Autodesk Inventor part; units mm, degrees
ref_plane "WeldJoint" through (0, 0, -10) normal (0.5, -0.866, 0) x (0, 0, 1)
ref_plane "Inlet_Clock_Angle_plane" through (0, 0, -10) normal (0, 1, 0) x (0, 0, 1)
ref_plane "Charging" through (0, 0, -10) normal (1, 0, 0) x (0, 0, 1)
sketch "Sketch13" plane through (0, 0, 0) normal (0, 0, 1) x (1, 0, 0)
  circle A0 centre (0, 0) radius 600 construction
  line L0 (0, 0) -> (0, -600)
  line L1 (0, 0) -> (-519.6152, -300)
  line L2 (0, 0) -> (600, 0)
  line L3 (0, 0) -> (0, -600)
  line L4 (0, 0) -> (0, -600)
  line L5 (0, 0) -> (534.6039, 272.3943)
  line L6 (0, 0) -> (0, 600)
  dimension "d53" = 1200
  dimension "d55" = 0
  dimension "d98" = 180
  dimension "d99" = 240
  dimension "d100" = 63
  dimension "d101" = 90
ref_plane "WeldJoint" through (0, 0, -10) normal (0.5, -0.866, 0) x (0, 0, 1)
ref_plane "Inlet_Clock_Angle_plane" through (0, 0, -10) normal (0, 1, 0) x (0, 0, 1)
ref_plane "Charging" through (0, 0, -10) normal (1, 0, 0) x (0, 0, 1)
ref_plane "Accsess" through (0, 0, -10) normal (1, 0, 0) x (0, 0, 1)
sketch "Sketch14" plane through (0, 0, -10) normal (0.5, -0.866, 0) x (0, 0, 1)
  line L0 (1710, 594) -> (10, 594)
  line L1 (10, 594) -> (10, 600)
  line L2 (10, 600) -> (1710, 600)
  line L3 (1710, 600) -> (1710, 594)
  line L4 (10, 0) -> (1710, 0)
  line L5 (10, 600) -> (-20, 600) construction
  line L6 (10, 594) -> (-20, 594) construction
  arc A0 (-20, 594) -> (-109.2789, 539.0476) centre (-20, 494) ccw construction
  arc A1 (-109.2789, 539.0476) -> (-234, 15) centre (929.3202, 15) ccw construction
  line L7 (-234, 15) -> (-234, 0) construction
  line L8 (10, 0) -> (-234, 0) construction
  arc A2 (-20, 600) -> (-114.6356, 541.7504) centre (-20, 494) ccw construction
  arc A3 (-114.6356, 541.7504) -> (-240, 15) centre (929.3202, 15) ccw construction
  line L9 (-240, 15) -> (-240, 0) construction
  line L10 (-234, 0) -> (-240, 0) construction
  line L11 (1710, 594) -> (1740, 594)
  line L12 (1710, 600) -> (1740, 600)
  line L13 (1710, 0) -> (1954, 0) construction
  line L14 (1960, 0) -> (1960, 15) construction
  arc A4 (1960, 15) -> (1834.6356, 541.7504) centre (790.6798, 15) ccw construction
  arc A5 (1834.6356, 541.7504) -> (1740, 600) centre (1740, 494) ccw construction
  line L15 (1954, 0) -> (1954, 15) construction
  line L16 (1954, 0) -> (1960, 0) construction
  arc A6 (1954, 15) -> (1829.2789, 539.0476) centre (790.6798, 15) ccw construction
  arc A7 (1829.2789, 539.0476) -> (1740, 594) centre (1740, 494) ccw construction
  line L17 (-160.8038, 520) -> (-540, 520)
  line L18 (-540, 520) -> (-540, 440)
  line L19 (-540, 440) -> (-160.8038, 440)
  line L20 (-160.8038, 440) -> (-160.8038, 520)
  line L21 (1960, 15) -> (1990, 15) construction
  line L22 (1990, 15) -> (1990, 0) construction
  line L23 (1990, 0) -> (1960, 0) construction
  line L24 (-540, 600) -> (-540, 520)
  line L25 (-540, 600) -> (-534, 600)
  line L26 (-534, 600) -> (-534, 520)
  line L27 (-120.3984, 533.7757) -> (-168.7178, 421.6324)
  line L28 (-160.8038, 520) -> (-126.334, 520)
  line L29 (-109.2789, 539.0476) -> (-114.6356, 541.7504)
  line L30 (-120.3984, 533.7757) -> (-116.5468, 542.7148) construction
  line L31 (-116.5468, 542.7148) -> (-114.6356, 541.7504) construction
  line L32 (-540, 600) -> (-540, 600)
  line L33 (-540, 600) -> (-540, 440)
  line L34 (-540, 440) -> (-540, 440)
  line L35 (1355, 600) -> (1265, 600)
  line L36 (1265, 600) -> (1265, 700)
  line L37 (1265, 700) -> (1355, 700)
  line L38 (1355, 700) -> (1355, 600)
  point P0 (10, 597)
  point P1 (-144.5581, 477.7041)
  point P2 (1310, 700)
  dimension "d59" = 1700
  dimension "d60" = 6
  dimension "d61" = 1200
  dimension "d82" = 100
  dimension "d83" = 30
  dimension "d86" = 80
  dimension "d87" = 30
  dimension "d91" = 15
  dimension "d92" = 20
  dimension "d93" = 250
  dimension "d94" = 30
  dimension "d103" = 413.666
  dimension "d104" = 23.31
  dimension "d105" = 122.1101
  dimension "d107" = 9.7336
  dimension "d108" = 880
  dimension "d109" = 0
  dimension "d110" = 2530
  dimension "d111" = 300
  dimension "d112" = 100
  dimension "d113" = 90
  dimension "d114" = 1850
  dimension "d115" = 1300
  dimension "d116" = 80
revolve "Revolution2" add sketch "Sketch14" angle 359.9 about axis through (0, 0, 0) along (0, 0, 1) contours L0 L1 L2 L3
sketch "Sketch AnglePlane_InletPipe" plane through (0, 0, -10) normal (0, 1, 0) x (0, 0, 1)
  line L0 (10, -600) -> (10, 600)
  line L1 (10, 0) -> (1310, 0)
  line L2 (1310, 0) -> (1310, 600)
  line L3 (1310, 600) -> (10, 600)
  line L4 (10, 600) -> (10, 0)
  point P0 (10, -519.6152)
  point P1 (10, -520.138)
  dimension "d63" = 1200
  dimension "d64" = 90
  dimension "frd_hght" = 1300
ref_plane "InletPipe_AnglePlane" through (0, 0, 1300) normal (1, 0, 0) x (0, 1, 0)
sketch "Sketch16" plane through (0, 0, 1300) normal (1, 0, 0) x (0, 1, 0)
  circle A0 centre (0, 0) radius 45.5
  point P0 (0, -1300)
  point P1 (0, 0)
  point P2 (0, 0)
  point P3 (0, 0)
  dimension "d66" = 91
extrude "Extrusion7" cut sketch "Sketch16" along normal through all
ref_plane "Work Plane16" through (0, 0, 0) normal (0, -1, 0) x (1, 0, 0)
sketch "Sketch17" plane through (0, 0, 0) normal (0, -1, 0) x (1, 0, 0)
  circle A0 centre (0, 416) radius 266
  line L0 (0, 150) -> (-495.5727, 150)
  point P0 (0, 0)
  dimension "d69" = 532
  dimension "d71" = 150
extrude "Extrusion8" cut sketch "Sketch17" along normal through all
sketch "ChargingAngleSketch19" plane through (0, 0, -10) normal (1, 0, 0) x (0, 0, 1)
  line L0 (10, 0) -> (963.5898, 0)
  line L1 (963.5898, 0) -> (1310, 600)
  line L2 (1310, 600) -> (10, 600)
  line L3 (10, 600) -> (10, 0)
  dimension "d74" = 1300
  dimension "d76" = 1200
  dimension "d77" = 60
ref_plane "Work Plane18" through (0, 0, 953.5898) normal (0, -0.866, 0.5) x (1, 0, 0)
sketch "Sketch20" plane through (0, 0, 953.5898) normal (0, -0.866, 0.5) x (1, 0, 0)
  line L0 (-104, 0) -> (104, 0)
  line L1 (104, 0) -> (104, 122)
  line L2 (104, 122) -> (-104, 122)
  line L3 (-104, 122) -> (-104, 0)
  point P0 (0, -825.833)
  point P1 (0, 0)
  point P2 (0, 0)
  point P3 (0, 0)
  point P4 (0, 0)
  dimension "d78" = 208
  dimension "d79" = 122
extrude "Charging hole" cut sketch "Sketch20" along normal through all
sketch "Sketch1" plane through (0, -1700, 0) normal (0, 0, 1) x (1, 0, 0)
  line L0 (520.8574, 1294.7565) -> (520.8574, 1435.6299)
  line L1 (728.7425, 1435.6299) -> (728.7425, 1294.7565)
  line L2 (532.8574, 1424.7204) -> (532.8574, 1307.9421)
  line L3 (716.7425, 1307.9421) -> (716.7425, 1424.7204)
  line L4 (624.7999, 682) -> (624.7999, 150) construction
  line L5 (350.7548, 416) -> (898.8451, 416) construction
  line L6 (1728.1139, 1564.2642) -> (1182.3519, -339.0339)
  line L7 (1182.3519, -339.0339) -> (0, 0)
  line L8 (0, 0) -> (545.762, 1903.2982)
  line L9 (545.762, 1903.2982) -> (1728.1139, 1564.2642)
  line L10 (1728.1139, 1564.2642) -> (0, 0) construction
  line L11 (1182.3519, -339.0339) -> (545.762, 1903.2982) construction
  line L12 (0, 0) -> (1279.5683, 0)
  line L13 (0, 1700) -> (0, 0)
  line L14 (0, 0) -> (3747.7583, 0)
  line L15 (0, 1700) -> (3747.7583, 1700)
  line L16 (3747.7583, 1700) -> (3747.7583, 0)
  ellipse E0 centre (624.7999, 416) end of major axis (624.7999, 150) minor radius 279
  line L17 (509.8574, 1445.5785) -> (509.8574, 1282.5939)
  line L18 (739.7425, 1282.5939) -> (739.7425, 1445.5785)
  point P0 (864.0569, 782.1321)
  point P1 (1516.7112, 1300)
  point P2 (1607.2885, 1300)
  point P3 (1595.2885, 1300)
  point P4 (1528.7112, 1300)
  point P5 (1254.7469, 1700)
  point P6 (487.4672, 1700)
  point P7 (729.8034, 1432.112)
  point P8 (519.7965, 1432.112)
  point P9 (520.8574, 1432.2183)
  point P10 (728.7425, 1432.2183)
  point P11 (1618.2885, 1300)
  point P12 (1505.7112, 1300)
  dimension "d0" = 12
  dimension "d10" = 12
  dimension "d13" = 279
  dimension "d15" = 11
  dimension "d16" = 11
  dimension "d17" = 11
  dimension "d3" = 532
  dimension "d4" = 548.0902
  dimension "d6" = 1980
  dimension "d8" = 1230
  dimension "d9" = 16
  dimension "d14" = 12
equation "\"BendRadius\" = Thickness"
equation "\"BendReliefWidth\" = Thickness"
equation "\"BendReliefDepth\" = 0.5 * Thickness"
equation "\"CornerReliefSize\" = 4 * Thickness"
equation "\"MinimumRemnant\" = 2 * Thickness"
equation "\"TransitionRadius\" = BendRadius"
equation "\"JacobiRadiusSize\" = BendRadius"
equation "\"GapSize\" = Thickness"
equation "\"InletPipe_horisont_angle\" = 0"
equation "\"ChargingHatch_width\" = 208"
equation "\"ChargingHatch_hight\" = 122"
equation "\"AccsessHatch_ClockAngle\" = 0"
equation "\"ChargingHatch_ClockAgnle\" = 180deg"
equation "\"InletPipe_Clock_angle\" = 90deg"
equation "\"OutletPipe_ClockAngle\" = 63deg"
equation "\"WeldJoint_ClockAgnle\" = 240deg"
equation "\"Legs_Tube_lenght\" = 413.666"
equation "\"Legs_Upper_plate_lenght\" = 122.11007"
properties part number "PRS 0101 main shell D1200" material "Steel"
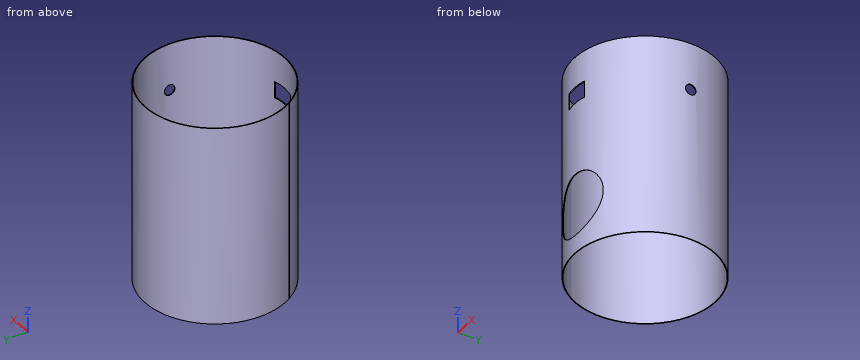
Read the model definition and answer for the solid it produces. Units are mm, in the model's axes. Coordinates: 2 decimals unless noted, no trailing zeros. Loops run counter-clockwise (first coordinate to the right, second up) from the corner with the lowest first, then second, coordinate; pieces in that order, holes last. Notation, with made-up numbers: (60.25, -37.5) - (70.25, -37.5) arc R24 ccw to (70.25, -11.5) - close; hole circle Ø1 at (61, -19). An arc over 180 degrees is marked (long way). Answer in a Markdown table with one row per item.
1. Find section A-A, the plane z = 1391. Write down the section's boundary in (x, y).
Conclusion:
| item | result |
|---|---|
| outline | (-520.14, -299.09) - (-514.94, -296.1) arc R594 cw (long way) to (104, -584.82) - (104, -590.92) arc R600 ccw (long way) to start; (-519.62, -300) arc R600 ccw to (-104, -590.92) - (-104, -584.82) arc R594 cw to (-514.42, -297) - close |
2. Find section D-D, the plane x = 197. Write down the section's boundary in (y, z), then the cut area to 3 significant figures.
Conclusion:
| item | result |
|---|---|
| outline | (-566.74, 0) - (-560.38, 0) - (-560.38, 237.26) - (-566.74, 237.26) - close; (-566.74, 594.74) - (-560.38, 594.74) - (-560.38, 1700) - (-566.74, 1700) - close; (560.38, 0) - (566.74, 0) - (566.74, 1700) - (560.38, 1700) - close |
| area | 19,300 mm² |
3. Find section B-B, the plane x = -60. Write down the section's boundary in (y, z).
Conclusion:
| item | result |
|---|---|
| outline | (-596.99, 0) - (-590.96, 0) - (-590.96, 156.86) - (-596.99, 156.86) - close; (-596.99, 675.14) - (-590.96, 675.14) - (-590.96, 1294.78) - (-596.99, 1298.26) - close; (-596.99, 1439.14) - (-590.96, 1435.66) - (-590.96, 1700) - (-596.99, 1700) - close; (590.96, 0) - (596.99, 0) - (596.99, 1700) - (590.96, 1700) - close |
4. Find section C-C, the plane y = -234. Write down the section's boundary in (x, z).
Conclusion:
| item | result |
|---|---|
| outline | (-552.49, 0) - (-545.97, 0) - (-545.97, 1700) - (-552.49, 1700) - close; (545.97, 0) - (552.49, 0) - (552.49, 1700) - (545.97, 1700) - close |
5. Given pin 1 (5 mm diameter, centred on y = 459, z = 1482.5, fed in from -X); pin 2 (10 mm diameter, centred on x = 241, z = 1111.5, fed in from -Y); pin 3 (1 mm diameter, centred on x = 225, z = 294.5, fed in from +Y), each flat-ended and moving along its own axis, determine where each tip first touches the part or whether it passes through.
Conclusion:
| item | result |
|---|---|
| pin 1 | stops at x = -389.37 |
| pin 2 | stops at y = -551.64 |
| pin 3 | stops at y = 556.42 |
6. Straight lines are drawn through the part: line 1 (X direction, y = 0, z = 822.5); line 2 (Z direction, x = 597, y = 0); line 3 (Y direction, x = 0, z = 416). For each, find the intervals that lie inside material, in ascending order.
Conclusion:
| item | result |
|---|---|
| line 1 | x = -600 to -594, 594 to 600 |
| line 2 | z = 0 to 1254.5, 1345.5 to 1700 |
| line 3 | y = 594 to 600 |
